Source: CAD feature listing. Evaluate the final solid. Frame: model axes, mm. A direction names the side the tool comes from. Give positions to 0.01 mm unless a question says otherwise; leave off trailing zeros. Write each loop counter-clockwise with the first axis right and the second up, starting at its lowest first coordinate (ties: lowest second). Pieces come first, ordered by that corner, then holes. Notation, with made-up numbers: M 54.5,83 L 87.5,83 A36 cw 87.5,119 Z; hole C -6,30.5 d7. An arc over 180 degrees is marked long. Return JSON: item names as keys, results as strings.
```python
from build123d import *

# Parameters (mm, degrees)
F1_DEPTH = 98.425
F2_R     = 1.778
F3_DEPTH = 25.4


with BuildPart() as f1:
    # F0 (on Top) → F1 (new body)
    with BuildSketch(Plane.XY):
        Polygon((6.35, 25.4), (6.35, 15.875), (12.7, 15.875), (12.7, 34.925), (6.35, 34.925), align=None)
        Polygon((0, 25.4), (0, 0), (6.35, 0), (6.35, 15.875), (6.35, 25.4), align=None)
    extrude(amount=F1_DEPTH)

    # F2 (on face) → F3 (cut)
    with BuildSketch(Plane.YZ.offset(6.35)):
        with Locations((7.9375, 73.025)):
            Circle(F2_R)
        with Locations((7.9375, 49.2125)):
            Circle(F2_R)
        with Locations((7.9375, 25.4)):
            Circle(F2_R)
    extrude(amount=-F3_DEPTH, mode=Mode.SUBTRACT)


solid = f1.part
```
1) Cut plane D-D, the plane x = 11.75. Return the cut outline in (y, z) (3 decimals), then the cut area to 4 significant figures.
Numbers:
{"outline": "M 15.875,0 L 34.925,0 L 34.925,98.425 L 15.875,98.425 Z", "area": "1,875 mm²"}
2) Contact query for flat-ended pins moving along their axis: pin 1 Ø3 at (x, z) = (2, 43) entering from +Y; pin 2 Ø1.9 at (x, z) = (8, 26) entering from -Y (3 decimals); pin 3 Ø8 at (y, z) = (7.5, 31) entering from +X. Output: stop coordinate, or through.
Numbers:
{"pin 1": "stops at y = 25.4", "pin 2": "stops at y = 15.875", "pin 3": "stops at x = 6.35"}
3) Cut plane C-C, the plane x = 2.75. Return the cut outline in (y, z) (1 decimal).
Numbers:
{"outline": "M 0,0 L 25.4,0 L 25.4,98.4 L 0,98.4 Z; hole C 7.9,25.4 d3.6; hole C 7.9,49.2 d3.6; hole C 7.9,73 d3.6"}
4) Cut plane B-B, the plane y = 8. Return the cut outline in (x, z) (3 decimals), then the cut area to 3 significant figures.
Numbers:
{"outline": "M 0,0 L 6.35,0 L 6.35,23.623 L 0,23.623 Z; M 0,27.177 L 6.35,27.177 L 6.35,47.436 L 0,47.436 Z; M 0,50.989 L 6.35,50.989 L 6.35,71.248 L 0,71.248 Z; M 0,74.802 L 6.35,74.802 L 6.35,98.425 L 0,98.425 Z", "area": "557 mm²"}
5) Draft query along Z for faces 4 (the face through (0, 13, 49)), 5 (the face through (6, 18, 98.425)), 6 (the face through (3.219, 7.706, 50.975)). Return one class per face: released by +Z, released by -Z, zero draft, split by the parting line, or undercut.
Numbers:
{"face 4": "zero draft", "face 5": "released by +Z", "face 6": "undercut"}
6) Set-up query: faces 1 (the face through (6.35, 6, 49)), 2 (the face through (3, 0, 49)), 3 (the face through (3, 25.4, 49)). Return all of +Z, -Z, +X, -X, +Y, -Y with unobstructed straight access to the full face (end or side cutting, diameter ignored); none if empty.
Numbers:
{"face 1": "+Z, -Z, +X, -Y", "face 2": "+Z, -Z, +X, -X, -Y", "face 3": "+Z, -Z, -X, +Y"}
7) Line query: line 1 (X direction, y = 12, z = 58.5); line 2 (Y direction, x = 4, z = 10.5); line 3 (Y direction, x = 10.25, z = 22) (3 decimals). Output: solid intervals per line, ascending. Write a range as [from, to].
Numbers:
{"line 1": "x = [0, 6.35]", "line 2": "y = [0, 25.4]", "line 3": "y = [15.875, 34.925]"}
